```python
from build123d import *

# Parameters (mm, degrees)
SKETCH_1_W               = 36
SKETCH_1_H               = 9.5
EXTRUDE_1_DEPTH          = 3
CUT_EXTRUDE_1_DEPTH      = 20.559204994
CUT_EXTRUDE_1_DEPTH_BACK = 20.559204994
SKETCH_2_R               = 4
CUT_EXTRUDE_2_DEPTH      = 20.559204994
CUT_EXTRUDE_2_DEPTH_BACK = 1
SKETCH_3_R               = 4
SKETCH_4_R               = 3
CUT_EXTRUDE_3_DEPTH      = 20.275956526
CHAMFER_1_SIZE           = 2


with BuildPart() as part:
    # 草图1 → 凸台-拉伸1 (new, symmetric)
    with BuildSketch(Plane.XY):
        Rectangle(SKETCH_1_W, SKETCH_1_H)
    extrude(amount=EXTRUDE_1_DEPTH, both=True)

    # 草图2 → 切除-拉伸1 (cut, two sides: drawn at the far end of the back side and taken through both)
    with BuildSketch(Plane.XY.offset(3).offset(-CUT_EXTRUDE_1_DEPTH_BACK)):
        with Locations((-13, 0)):
            Circle(SKETCH_2_R)
    extrude(amount=CUT_EXTRUDE_1_DEPTH + CUT_EXTRUDE_1_DEPTH_BACK, mode=Mode.SUBTRACT)

    # 草图3 → 切除-拉伸2 (cut, two sides: drawn at the far end of the back side and taken through both)
    with BuildSketch(Plane.XY.offset(3).offset(-CUT_EXTRUDE_2_DEPTH_BACK)):
        with Locations(Location((13, 0, 0), (0, 0, 180))):
            Circle(SKETCH_3_R)
    extrude(amount=CUT_EXTRUDE_2_DEPTH + CUT_EXTRUDE_2_DEPTH_BACK, mode=Mode.SUBTRACT)

    # 草图4 → 切除-拉伸3 (cut, through all)
    with BuildSketch(Plane.XY.offset(2)):
        with Locations((13, 0)):
            Circle(SKETCH_4_R)
    extrude(amount=-CUT_EXTRUDE_3_DEPTH, mode=Mode.SUBTRACT)

    # 倒角1
    chamfer_1_edges = [part.edges().sort_by_distance(p)[0] for p in [
        (18, -4.75, 0),
        (-18, -4.75, 0),
        (-18, 4.75, 0),
        (18, 4.75, 0),
    ]]
    chamfer(chamfer_1_edges, length=CHAMFER_1_SIZE)


solid = part.part
```
Geometry check sheet. Reference: the model listing, model coordinates, mm. A direction names the side the tool comes from. Round coordinates to 2 decimals unless told otherwise and drop trailing zeros. Write each loop counter-clockwise with the first axis right and the second up, starting at its lowest first coordinate (ties: lowest second). Pieces come first, ordered by that corner, then holes. Notation, with made-up numbers: (75, 37.5) -> (86, 37.5) arc R12 ccw to (86, 56.5) -> close; hole circle Ø7 at (85, -37). An arc over 180 degrees is marked (long way). Put each result on its own line as item: value.
1) Cross-section at B-B, the plane y = 0. Enter the section's corners in (x, z), plus the area to 3 significant figures.
Recorded:
outline: (-18, -3) -> (-17, -3) -> (-17, 3) -> (-18, 3) -> close; (-9, -3) -> (10, -3) -> (10, 2) -> (9, 2) -> (9, 3) -> (-9, 3) -> close; (16, -3) -> (18, -3) -> (18, 3) -> (17, 3) -> (17, 2) -> (16, 2) -> close
area: 130 mm2
2) Cross-section at C-C, the plane y = -3.5. Enter the section's corners in (x, z), plus the area to 3 significant figures.
Recorded:
outline: (-17.25, -3) -> (-14.94, -3) -> (-14.94, 3) -> (-17.25, 3) -> close; (-11.06, -3) -> (17.25, -3) -> (17.25, 3) -> (14.94, 3) -> (14.94, 2) -> (11.06, 2) -> (11.06, 3) -> (-11.06, 3) -> close
area: 180 mm2
3) Thickness scan on probe 1 along X at (y, z) = (-3.5, 2.7); probe 2 along Y at (x, z) = (13, -0.8); probe 3 along X at (y, z) = (-0.75, 1.35). Record the ranges inside material, lowest first. Write a range as from..to.
Recorded:
probe 1: x = -17.25..-14.94, -11.06..11.06, 14.94..17.25
probe 2: y = -4.75..-3, 3..4.75
probe 3: x = -18..-16.93, -9.07..10.1, 15.9..18
4) Cross-section at D-D, the plane z = 0.05. Enter the section's corners in (x, y).
Recorded:
outline: (-18, -2.75) -> (-16, -4.75) -> (16, -4.75) -> (18, -2.75) -> (18, 2.75) -> (16, 4.75) -> (-16, 4.75) -> (-18, 2.75) -> close; hole circle Ø8 at (-13, 0); hole circle Ø6 at (13, 0)
5) Cross-section at A-A, the plane x = -13. Enter the section's corners in (y, z).
Recorded:
outline: (-4.75, -3) -> (-4, -3) -> (-4, 3) -> (-4.75, 3) -> close; (4, -3) -> (4.75, -3) -> (4.75, 3) -> (4, 3) -> close
6) Access from +Z, -Z, +X, -X, +Y, -Y to the whole of each face (thin tool, end or side, straight path). Record for faces 1 (the face through (10, 0, 0)), 2 (the face through (12, -3, 2)).
Recorded:
face 1: +Z, -Z
face 2: +Z
